Input: part model. Units: mm. Frame: model coordinates. A direction names the side the tool comes from. Round coordinates to 2 decimals unless told otherwise and drop trailing zeros. Write each loop counter-clockwise with the first axis right and the second up, starting at its lowest first coordinate (ties: lowest second). Pieces come first, ordered by that corner, then holes. Notation, with made-up numbers: (-36, 57.5) -> (-1, 57.5) arc R16 ccw to (-1, 86.5) -> close; hole circle Ø10 at (70.25, -2.5). An arc over 180 degrees is marked (long way). Write item = value, one per line. Start each with the question number.
Autodesk Inventor part; units mm, degrees
ref_plane "YZ Plane" through (0, 0, 0) normal (1, 0, 0) x (0, 1, 0)
ref_plane "XZ Plane" through (0, 0, 0) normal (0, 1, 0) x (-1, 0, 0)
ref_plane "XY Plane" through (0, 0, 0) normal (0, 0, 1) x (1, 0, 0)
sketch "Sketch1" plane through (0, 0, 0) normal (0, 1, 0) x (-1, 0, 0)
  circle A0 centre (-26.3449, -3.1424) radius 2
  arc A1 (-35.0949, -0.1424) -> (-17.5949, -0.1424) centre (-26.3449, -0.1424) ccw
  arc A2 (17.4051, -0.1424) -> (34.9051, -0.1424) centre (26.1551, -0.1424) ccw
  circle A3 centre (26.1551, -3.1424) radius 2
  circle A4 centre (-26.3449, -3.1424) radius 2
  circle A5 centre (26.1551, -3.1424) radius 2
  circle A6 centre (26.1551, -0.1424) radius 8.75
  circle A7 centre (-26.3449, -0.1424) radius 8.75
  line L0 (-35.0949, -0.1424) -> (-17.5949, -0.1424)
  line L1 (17.4051, -0.1424) -> (34.9051, -0.1424)
  circle A8 centre (-26.3449, -3.1424) radius 5.5
  circle A9 centre (26.1551, -3.1424) radius 5.5
  line L2 (-26.3449, -8.6424) -> (26.1551, -8.6424)
  line L3 (-26.3449, 2.3576) -> (26.1551, 2.3576)
  point P0 (0, 0)
  point P1 (-0.1898, -0.0949)
  dimension "d0" = 11
  dimension "d1" = 11
extrude "Extrusion1" add sketch "Sketch1" along normal blind 20 contours L2 A8 L0 A1 | A1 A7 L3 A6 A2 L2 | A7 L0 A8 L3 | A8 L0 | L0 A8 | A2 L1 A9 L2 | L3 A9 L1 A6 | A9 L1 | A9 L1 picked at (-18.8837, -1.0963) picked at (-20.7697, 1.0381) picked at (18.6638, -1.1758) picked at (20.5799, 1.0381)
sketch "Sketch2" plane through (0, 20, 0) normal (0, 1, 0) x (1, 0, 0)
  circle A0 centre (-26.1551, 3.1424) radius 2
  circle A1 centre (26.3449, 3.1424) radius 2
  circle A2 centre (-26.1551, 3.1424) radius 5.5
  circle A3 centre (26.3449, 3.1424) radius 5.5
  line L0 (26.3449, 8.6424) -> (-26.1551, 8.6424)
  line L1 (-20.6551, 8.6424) -> (-20.6551, -2.3576)
  line L2 (-26.1551, -2.3576) -> (26.3449, -2.3576)
  line L3 (20.8449, 8.6424) -> (20.8449, -2.3576)
  line L4 (-26.1551, 8.6424) -> (-20.6551, 8.6424)
  line L5 (-26.1551, -2.3576) -> (-20.6551, -2.3576)
  line L6 (20.8449, 8.6424) -> (26.3449, 8.6424)
  line L7 (20.8449, -2.3576) -> (26.3449, -2.3576)
  point P0 (0, 0)
extrude "Extrusion2" cut sketch "Sketch2" against normal blind 10 contours A2 | L1 L2 A2 | A2 L0 L1 | L0 A3 L3 | L3 A3 L2 | A3
sketch "Sketch4" plane through (0, 20, 0) normal (0, 1, 0) x (1, 0, 0)
  line L0 (20.8449, 8.6424) -> (-20.6551, 8.6424)
  line L1 (-20.6551, -2.3576) -> (20.8449, -2.3576)
  line L2 (-20.6551, 8.6424) -> (20.8449, 8.6424)
  line L3 (20.8449, 8.6424) -> (20.8449, -2.3576)
  line L4 (20.8449, -2.3576) -> (-20.6551, -2.3576)
  line L5 (-20.6551, -2.3576) -> (-20.6551, 8.6424)
  line L6 (-20.6551, -2.3576) -> (20.8449, -2.3576)
  line L7 (20.8449, -2.3576) -> (20.8449, -17.3636)
  line L8 (20.8449, -17.3636) -> (-20.6551, -17.3636)
  line L9 (-20.6551, -17.3636) -> (-20.6551, -2.3576)
  line L10 (9.5949, -22.8636) -> (-9.4051, -22.8636)
  line L11 (-9.4051, -22.8636) -> (-9.4051, -11.8636)
  line L12 (-9.4051, -11.8636) -> (9.5949, -11.8636)
  line L13 (9.5949, -11.8636) -> (9.5949, -22.8636)
  line L14 (9.5949, -22.8636) -> (-9.4051, -11.8636) construction
  line L15 (-9.4051, -22.8636) -> (9.5949, -11.8636) construction
  circle A0 centre (-4.9051, -20.3636) radius 2
  circle A1 centre (5.0949, -20.3636) radius 2
  point P0 (0, 0)
  point P1 (-9.4051, -17.3636)
  point P2 (9.5949, -17.3636)
  dimension "d27" = 19
  dimension "d28" = 11
  dimension "d29" = 4
  dimension "d30" = 3
  dimension "d31" = 4.5
  dimension "d32" = 4
  dimension "d33" = 3
  dimension "d34" = 4.5
  dimension "d37" = 20.506
extrude "Extrusion5" add sketch "Sketch4" along normal blind 4.56
sketch "Sketch5" plane through (0, 24.56, 0) normal (0, 1, 0) x (1, 0, 0)
  line L0 (-9.4051, -22.8636) -> (9.5949, -22.8636)
  line L1 (9.5949, -17.3636) -> (20.8449, -17.3636)
  line L2 (-9.4051, -22.8636) -> (9.5949, -22.8636)
  line L3 (9.5949, -22.8636) -> (9.5949, -17.3636)
  line L4 (9.5949, -17.3636) -> (-9.4051, -17.3636)
  line L5 (-9.4051, -17.3636) -> (-9.4051, -22.8636)
  line L6 (-0.5051, -27.3636) -> (0.6949, -27.3636)
  line L7 (0.6949, -27.3636) -> (0.6949, -18.3636)
  line L8 (0.6949, -18.3636) -> (-0.5051, -18.3636)
  line L9 (-0.5051, -18.3636) -> (-0.5051, -27.3636)
  line L10 (-0.5051, -27.3636) -> (0.6949, -18.3636) construction
  line L11 (0.6949, -27.3636) -> (-0.5051, -18.3636) construction
  point P0 (0, 0)
  point P1 (0.0949, -22.8636)
  dimension "d41" = 1.2
extrude "Extrusion6" cut sketch "Sketch5" against normal blind 4.56 contours L9 L8 L7 L0 | L0 L7 L6 L9
sketch "Sketch6" plane through (0, 24.56, 0) normal (0, 1, 0) x (1, 0, 0)
  line L0 (26.3449, -2.3576) -> (20.8449, -2.3576)
  arc A0 (26.3449, -2.3576) -> (26.3449, 8.6424) centre (26.3449, 3.1424) ccw
  line L1 (20.8449, 8.6424) -> (26.3449, 8.6424)
  line L2 (20.8449, -2.3576) -> (20.8449, 8.6424)
  circle A1 centre (26.3449, 3.1424) radius 2
  line L3 (-20.6551, -2.3576) -> (-26.1551, -2.3576)
  line L4 (-20.6551, 8.6424) -> (-20.6551, -2.3576)
  line L5 (-26.1551, 8.6424) -> (-20.6551, 8.6424)
  arc A2 (-26.1551, 8.6424) -> (-26.1551, -2.3576) centre (-26.1551, 3.1424) ccw
  circle A3 centre (-26.1551, 3.1424) radius 2
  circle A4 centre (5.0949, -20.3636) radius 2
  circle A5 centre (-4.9051, -20.3636) radius 2
  line L6 (-0.5051, -22.8636) -> (-0.5051, -18.3636)
  line L7 (-0.5051, -18.3636) -> (0.6949, -18.3636)
  line L8 (0.6949, -18.3636) -> (0.6949, -22.8636)
  line L9 (0.6949, -22.8636) -> (9.5949, -22.8636)
  line L10 (9.5949, -22.8636) -> (9.5949, -17.3636)
  line L11 (9.5949, -17.3636) -> (20.8449, -17.3636)
  line L12 (20.8449, -17.3636) -> (20.8449, 8.6424)
  line L13 (20.8449, 8.6424) -> (-20.6551, 8.6424)
  line L14 (-20.6551, 8.6424) -> (-20.6551, -17.3636)
  line L15 (-20.6551, -17.3636) -> (-9.4051, -17.3636)
  line L16 (-9.4051, -17.3636) -> (-9.4051, -22.8636)
  line L17 (-9.4051, -22.8636) -> (-0.5051, -22.8636)
  line L18 (20.8449, -2.3576) -> (9.5949, -17.3636)
  line L19 (9.5949, -17.3636) -> (-9.4051, -17.3636)
  line L20 (20.8449, -17.3636) -> (20.8449, 8.6424)
  line L21 (-9.4051, -17.3636) -> (-20.6551, -2.3576)
  line L22 (-9.4051, -17.3636) -> (-20.6551, -17.3636)
  line L23 (-20.6551, -17.3636) -> (-20.6551, -2.3576)
  line L24 (20.8449, -17.3636) -> (9.5949, -17.3636)
  line L25 (20.8449, -17.3636) -> (20.8449, -2.3576)
  point P0 (0, 0)
extrude "Extrusion7" cut sketch "Sketch6" against normal blind 4.56 contours L12 L11 L18 | L15 L14 L21
properties part number "Servo holder long side"
1. Reachability of faces 4 (the flat face through (0, 20, 10)), 5 (the flat face through (-0.505, 22, 21)), 6 (the flat face through (9.595, 22, 20)), 7 (the flat face through (-9.405, 22, 20)), 8 (the flat face through (-24, 10, -3)) from +Z, -Z, +X, -X, +Y, -Y: full face, straight path, thin tool, end or side. Return the list, or none.
2. Section B-B (y = 22). Output: boundary loops of the cut face in (x, z).
3. Mould query, pull axis Z, two halves, no side actions, for faces 1 (the cylindrical face through (4.66, 22.25, 18.41)), 2 (the flat face through (-20.655, 17, -3)), 3 (the flat face through (5, 22, 22.864)). Classes: pulls with the +Z half, pulls with the -Z half, needs draft (parallel to the pull), parting line crosses it, or undercut.
4. Pin query (flat end, axial travel): P1, Ø2, axis at y = 23.5, z = 20, coming from the +X side; P2, Ø3, axis at y = 20.5, z = 10.5, coming from the +X side; P3, Ø9, axis at x = -27, z = -3.5, coming from the +Y side. Return the tip coordinate at first contact, or that it passes through.
5. Section A-A (x = -5). Output: boundary loops of the cut face in (y, z).
6. Line query: line 1 along Z through (x, y) = (-24, 5.25); line 2 along Y through (x, z) = (0, 3); line 3 along X through (y, z) = (23.5, -5). Output: solid intervals per line, ascending.
7. Section C-C (x = 8.5). Output: boundary loops of the cut face in (y, z).
8. Section D-D (y = 16.75). Output: boundary loops of the cut face in (x, z).
Check sheet entries:
q1.face_4 = +Z, +X, -X, -Y
q1.face_5 = +Z, +Y, -Y
q1.face_6 = +Z, +X, +Y, -Y
q1.face_7 = +Z, -X, +Y, -Y
q1.face_8 = +Z, -Z, -X, +Y
q2.outline = (-20.66, -8.64) -> (20.84, -8.64) -> (20.84, 2.36) -> (9.59, 17.36) -> (9.59, 22.86) -> (0.69, 22.86) -> (0.69, 18.36) -> (-0.51, 18.36) -> (-0.51, 22.86) -> (-9.41, 22.86) -> (-9.41, 17.36) -> (-20.66, 2.36) -> close; hole circle Ø4 at (-4.91, 20.36); hole circle Ø4 at (5.09, 20.36)
q3.face_1 = undercut
q3.face_2 = needs draft
q3.face_3 = pulls with the +Z half
q4.P1 = 9.59
q4.P2 = 15.87
q4.P3 = 10
q5.outline = (0, -8.64) -> (24.56, -8.64) -> (24.56, 18.37) -> (20, 18.37) -> (20, 2.36) -> (0, 2.36) -> close; (20, 22.36) -> (24.56, 22.36) -> (24.56, 22.86) -> (20, 22.86) -> close
q6.line_1 = -8.64 to 2.36
q6.line_2 = 20 to 24.56
q6.line_3 = -20.66 to 20.84
q7.outline = (0, -8.64) -> (24.56, -8.64) -> (24.56, 22.86) -> (20, 22.86) -> (20, 2.36) -> (0, 2.36) -> close
q8.outline = (-20.66, -8.64) -> (20.84, -8.64) -> (20.84, 2.36) -> (-20.66, 2.36) -> close
